Source: CAD feature listing. Evaluate the final solid. Frame: model axes, mm. Face numbers are marked on the shaded views. Give positions to 0.01 mm unless a question says otherwise; leave off trailing zeros. Order: outer loops, then holes, each group sorted by start corner. A loop starts at its lowest first (then second) coordinate and runs counter-clockwise, first axis right, second up. Notation, with made-up numbers: M 86,33.5 L 138,33.5 A18 ccw 138,56.5 Z; hole C 58,73.5 d5. An arc over 180 degrees is marked long. Return JSON: item names as keys, results as strings.
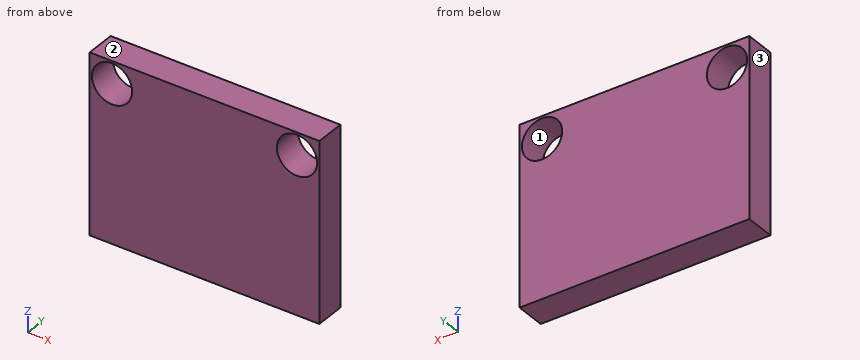
from build123d import *

# Parameters (mm, degrees)
BOSS_EXTRUDE1_OUTLINE_W = 154
BOSS_EXTRUDE1_OUTLINE_H = 120
BOSS_EXTRUDE1_DEPTH     = 20
SKETCH2_R               = 13.5
CUT_EXTRUDE3_DEPTH      = 144.975692393


# Read off the part's stored shape, not the designer's step: Boss-Extrude1
with BuildPart() as part:
    # Boss-Extrude1 outline → Boss-Extrude1 (new body)
    with BuildSketch(Plane(origin=(0, 0, 0), x_dir=(1, 0, 0), z_dir=(0, 1, 0))):
        with Locations((0, 60)):
            Rectangle(BOSS_EXTRUDE1_OUTLINE_W, BOSS_EXTRUDE1_OUTLINE_H)
    extrude(amount=BOSS_EXTRUDE1_DEPTH)

    # Sketch2 → Cut-Extrude3 (cut, through all)
    with BuildSketch(Plane.XZ):
        with Locations(Location((62, -15, 0), (0, 0, 270))):
            Circle(SKETCH2_R)
    cut_extrude3 = extrude(amount=-CUT_EXTRUDE3_DEPTH, mode=Mode.SUBTRACT)

    # Mirror1: Cut-Extrude3 across plane
    add(cut_extrude3.mirror(Plane(origin=(0, 0, 0), x_dir=(0, 0, 1), z_dir=(1, 0, 0))), mode=Mode.SUBTRACT)


solid = part.part
1. Section query A-A (x = 62). Return loops of the section in (y, z), then the cut area to 3 significant figures.
Evaluation:
{"outline": "M 0,-120 L 20,-120 L 20,-28.5 L 0,-28.5 Z; M 0,-1.5 L 20,-1.5 L 20,0 L 0,0 Z", "area": "1,860 mm^2"}
2. Draft query along X for the marked faces 1, 2 and 3. Return one class per face: pulls with the +X half, pulls with the -X half, needs draft (parallel to the pull), parting line crosses it, or undercut.
Evaluation:
{"face 1": "undercut", "face 2": "needs draft", "face 3": "pulls with the -X half"}
3. Section query C-C (y = 9.5). Return loops of the section in (x, z), then the cut area to 3 significant figures.
Evaluation:
{"outline": "M -77,-120 L 77,-120 L 77,0 L -77,0 Z; hole C -62,-15 d27; hole C 62,-15 d27", "area": "17,300 mm^2"}
4. Section query B-B (z = -15). Return loops of the section in (x, y).
Evaluation:
{"outline": "M -77,0 L -75.5,0 L -75.5,20 L -77,20 Z; M -48.5,0 L 48.5,0 L 48.5,20 L -48.5,20 Z; M 75.5,0 L 77,0 L 77,20 L 75.5,20 Z"}
5. Ray query, probe 1 along X at (y, z) = (11.75, -15); probe 2 along Z at (x, y) = (-62, 7); probe 3 along X at (y, z) = (16, -17). Return the intervals inside material, ascending.
Evaluation:
{"probe 1": "x = -77 to -75.5, -48.5 to 48.5, 75.5 to 77", "probe 2": "z = -120 to -28.5, -1.5 to 0", "probe 3": "x = -77 to -75.35, -48.65 to 48.65, 75.35 to 77"}
6. First-contact query: pin 1 (21.5 mm diameter, centred on x = 62, z = -15, fed in from +Y). Flat tip, straight axial feed; report the tip coordinate or a pass-through.
Evaluation:
{"pin 1": "passes through"}
